Can you work these out from the model? Positions are in its coordinate system, mm. A direction names the side the tool comes from. Give positions to 0.01 mm unless a question says otherwise; leave off trailing zeros. Write each loop counter-clockwise with the first axis right and the second up, starting at its lowest first coordinate (ties: lowest second). Pieces come first, ordered by that corner, then holes.
1. On a 3-axis mill with a long thin cutter (end or side, diameter ignored), from which of +Z, -Z, +X, -X, +Y, -Y can I reach the whole of each face in a straight line? I mean faces 1 (the flat face through (0, -9, 4)), 2 (the flat face through (10, 0, 4)). Say none if no direction works.
2. If I drill on probe 1 along X at (y, z) = (-9.6, -286) (3 decimals); probe 2 along X at (y, z) = (-4, -260), over which ranges is the centre line in solid material (lowest first)?
3. I'm going to push a flat-ended pin straight in: pin 1 (3.5 mm diameter, centred on y = 0, z = 260, fed in from -X). Where does the tip first touch, or does it pass through?
4. Thinking about a two-plate mould opening in Y: for faces 3 (the flat face through (-10, 0, 4)), 4 (the flat face through (0, 9, 4)), 5 (the flat face through (0, 10, 4)), 6 (the flat face through (9, 0, 4)), which applies, pulls with the +Y half, pulls with the -Y half, needs draft (parallel to the pull), parting line crosses it, or undercut?
5. Suppose I cut it at A-A (z = 90). Please give me the cut outline in (x, y), and give its area (3 significant figures).
```python
from build123d import *

# Parameters (mm, degrees)
SKETCH_1_W          = 20
SKETCH_1_H          = 20
SKETCH_1_W_2        = 18
SKETCH_1_H_2        = 18
EXTRUDE_1_DEPTH     = 310
SKETCH_2_R          = 2.025
SKETCH_2_R_2        = 3.05
CUT_EXTRUDE_1_DEPTH = 30
SKETCH_3_R          = 2.1
CUT_EXTRUDE_2_DEPTH = 30
SKETCH_4_R          = 2.05
CUT_EXTRUDE_3_DEPTH = 20


with BuildPart() as part:
    # 草图1 → 凸台-拉伸1 (new, symmetric)
    with BuildSketch(Plane.XY):
        Rectangle(SKETCH_1_W, SKETCH_1_H)
        Rectangle(SKETCH_1_W_2, SKETCH_1_H_2, mode=Mode.SUBTRACT)
    extrude(amount=EXTRUDE_1_DEPTH, both=True)

    # 草图2 → 切除-拉伸1 (cut)
    with BuildSketch(Plane(origin=(0, 10, 0), x_dir=(1, 0, 0), z_dir=(0, 1, 0))):
        with Locations(Location((-5, -286, 0), (0, 0, 270))):
            Circle(SKETCH_2_R)
        with Locations(Location((5, -286, 0), (0, 0, 270))):
            Circle(SKETCH_2_R)
        with Locations(Location((-5, -306, 0), (0, 0, 270))):
            Circle(SKETCH_2_R)
        with Locations(Location((5, -306, 0), (0, 0, 270))):
            Circle(SKETCH_2_R)
        with Locations(Location((0, -296, 0), (0, 0, 270))):
            Circle(SKETCH_2_R_2)
        with Locations((5, 306)):
            Circle(SKETCH_2_R)
        with Locations((5, 286)):
            Circle(SKETCH_2_R)
        with Locations((-5, 286)):
            Circle(SKETCH_2_R)
        with Locations((0, 296)):
            Circle(SKETCH_2_R_2)
        with Locations((-5, 306)):
            Circle(SKETCH_2_R)
    extrude(amount=-CUT_EXTRUDE_1_DEPTH, mode=Mode.SUBTRACT)

    # 草图3 → 切除-拉伸2 (cut)
    with BuildSketch(Plane(origin=(0, 10, 0), x_dir=(1, 0, 0), z_dir=(0, 1, 0))):
        with Locations(Location((0, 150, 0), (0, 0, 270))):
            Circle(SKETCH_3_R)
        with Locations(Location((0, 75, 0), (0, 0, 270))):
            Circle(SKETCH_3_R)
        with Locations(Location((0, 0, 0), (0, 0, 270))):
            Circle(SKETCH_3_R)
        with Locations(Location((0, -75, 0), (0, 0, 270))):
            Circle(SKETCH_3_R)
        with Locations(Location((0, -150, 0), (0, 0, 270))):
            Circle(SKETCH_3_R)
    extrude(amount=-CUT_EXTRUDE_2_DEPTH, mode=Mode.SUBTRACT)

    # 草图4 → 切除-拉伸3 (cut, symmetric)
    with BuildSketch(Plane(origin=(10, 0, 0), x_dir=(0, 0, -1), z_dir=(1, 0, 0))):
        with Locations((-300, 0)):
            Circle(SKETCH_4_R)
        with Locations((-280, 0)):
            Circle(SKETCH_4_R)
        with Locations((-260, 0)):
            Circle(SKETCH_4_R)
        with Locations((-240, 0)):
            Circle(SKETCH_4_R)
        with Locations((-220, 0)):
            Circle(SKETCH_4_R)
        with Locations((-200, 0)):
            Circle(SKETCH_4_R)
        with Locations((-180, 0)):
            Circle(SKETCH_4_R)
        with Locations((-160, 0)):
            Circle(SKETCH_4_R)
        with Locations((-140, 0)):
            Circle(SKETCH_4_R)
        with Locations((-120, 0)):
            Circle(SKETCH_4_R)
        with Locations((-100, 0)):
            Circle(SKETCH_4_R)
        with Locations((-80, 0)):
            Circle(SKETCH_4_R)
        with Locations((-60, 0)):
            Circle(SKETCH_4_R)
        with Locations((-40, 0)):
            Circle(SKETCH_4_R)
        with Locations((-20, 0)):
            Circle(SKETCH_4_R)
        Circle(SKETCH_4_R)
        with Locations((20, 0)):
            Circle(SKETCH_4_R)
        with Locations((40, 0)):
            Circle(SKETCH_4_R)
        with Locations((60, 0)):
            Circle(SKETCH_4_R)
        with Locations((80, 0)):
            Circle(SKETCH_4_R)
        with Locations((100, 0)):
            Circle(SKETCH_4_R)
        with Locations((120, 0)):
            Circle(SKETCH_4_R)
        with Locations((140, 0)):
            Circle(SKETCH_4_R)
        with Locations((160, 0)):
            Circle(SKETCH_4_R)
        with Locations((180, 0)):
            Circle(SKETCH_4_R)
        with Locations((200, 0)):
            Circle(SKETCH_4_R)
        with Locations((220, 0)):
            Circle(SKETCH_4_R)
        with Locations((240, 0)):
            Circle(SKETCH_4_R)
        with Locations((260, 0)):
            Circle(SKETCH_4_R)
        with Locations((280, 0)):
            Circle(SKETCH_4_R)
        with Locations((300, 0)):
            Circle(SKETCH_4_R)
    extrude(amount=CUT_EXTRUDE_3_DEPTH, both=True, mode=Mode.SUBTRACT)


solid = part.part
```
Checks:
1. face 1: +Z, -Z
1. face 2: +Z, -Z, +X, +Y, -Y
2. probe 1: x = -10 to -7.025, -2.975 to 2.975, 7.025 to 10
2. probe 2: x = -10 to -9, 9 to 10
3. pin 1: passes through
4. face 3: needs draft
4. face 4: undercut
4. face 5: pulls with the +Y half
4. face 6: undercut
5. outline: (-10, -10) - (10, -10) - (10, 10) - (-10, 10) - close; hole (-9, -9) - (9, -9) - (9, 9) - (-9, 9) - close
5. area: 76.0 mm2
